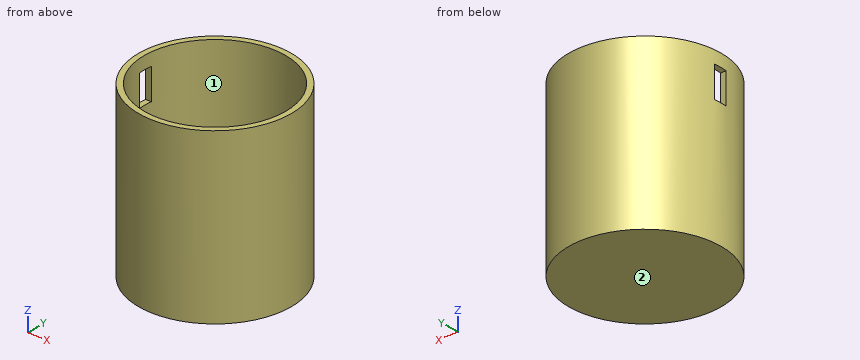
from build123d import *

# Parameters (mm, degrees)
F0_R     = 27
F0_R_2   = 25
F1_DEPTH = 60
F2_W     = 5
F2_H     = 11
F3_DEPTH = 25
F4_DEPTH = 30
F5_DEPTH = 2


with BuildPart() as f1:
    # F0 (on Top) → F1 (new body)
    with BuildSketch(Plane.XY):
        Circle(F0_R)
        Circle(F0_R_2, mode=Mode.SUBTRACT)
    extrude(amount=F1_DEPTH)

    # F2 (on Right) → F3 (cut)
    with BuildSketch(Plane.YZ):
        with Locations((0, 50)):
            Rectangle(F2_W, F2_H)
    extrude(amount=-F3_DEPTH, mode=Mode.SUBTRACT)

    # F2 (on Right) → F4 (cut)
    with BuildSketch(Plane.YZ):
        with Locations((0, 50)):
            Rectangle(F2_W, F2_H)
    extrude(amount=-F4_DEPTH, mode=Mode.SUBTRACT)

    # F0 (on Top) → F5 (join)
    with BuildSketch(Plane.XY):
        Circle(F0_R_2)
    extrude(amount=F5_DEPTH)


solid = f1.part
Check sheet for the modelled part. Datum: model origin and axes. Units: mm. Face numbers are marked on the shaded views. A direction names the side the tool comes from. Give positions to 0.01 mm unless a question says otherwise; leave off trailing zeros. Write each loop counter-clockwise with the first axis right and the second up, starting at its lowest first coordinate (ties: lowest second). Pieces come first, ordered by that corner, then holes. Notation, with made-up numbers: (71, -22) -> (104, -22) arc R17 cw to (104, 7) -> close; hole circle Ø6 at (41.5, -13). An arc over 180 degrees is marked (long way). Use one line per item in the form item = value. Start each with the question number.
1. Section check B-B (x = 0). Record the cut outline in (y, z), and give its area (3 significant figures).
2. Section check C-C (y = 23). Record the cut outline in (x, z), and give its area (3 significant figures).
3. Section check D-D (z = 48). Record the cut outline in (x, y), and give its area (3 significant figures).
4. Section check A-A (y = 0). Record the cut outline in (x, z).
5. Thickness scan on line 1 along X through (y, z) = (0, 20); line 2 along Z through (x, y) = (-18.5, 0.5). Record the ranges inside material, lowest first. Write a range as from..to.
6. Access from +Z, -Z, +X, -X, +Y, -Y to the whole of each face (thin tool, end or side, straight path). Record for the marked faces 1 and 2.
7. Go/stop test with flat-tipped pins: P1, Ø10, axis at y = 14.5, z = 53.5, coming from the +X side; P2, Ø15, axis at x = -9, y = 6, coming from the +Z side; P3, Ø10, axis at y = 7, z = 28.5, coming from the +X side. Record where each tip stops, or that it passes through.
Conclusion:
q1.outline = (-27, 0) -> (27, 0) -> (27, 60) -> (25, 60) -> (25, 2) -> (-25, 2) -> (-25, 60) -> (-27, 60) -> close
q1.area = 340 mm²
q2.outline = (-14.14, 0) -> (14.14, 0) -> (14.14, 60) -> (9.8, 60) -> (9.8, 2) -> (-9.8, 2) -> (-9.8, 60) -> (-14.14, 60) -> close
q2.area = 560 mm²
q3.outline = (-26.88, -2.5) arc R27 ccw (long way) to (-26.88, 2.5) -> (-24.87, 2.5) arc R25 cw (long way) to (-24.87, -2.5) -> close
q3.area = 317 mm²
q4.outline = (-27, 0) -> (27, 0) -> (27, 60) -> (25, 60) -> (25, 2) -> (-25, 2) -> (-25, 44.5) -> (-27, 44.5) -> close; (-27, 55.5) -> (-25, 55.5) -> (-25, 60) -> (-27, 60) -> close
q5.line_1 = -27..-25, 25..27
q5.line_2 = 0..2
q6.face_1 = +Z
q6.face_2 = -Z, +X, -X, +Y, -Y
q7.P1 = 25.27
q7.P2 = 2
q7.P3 = 26.93
